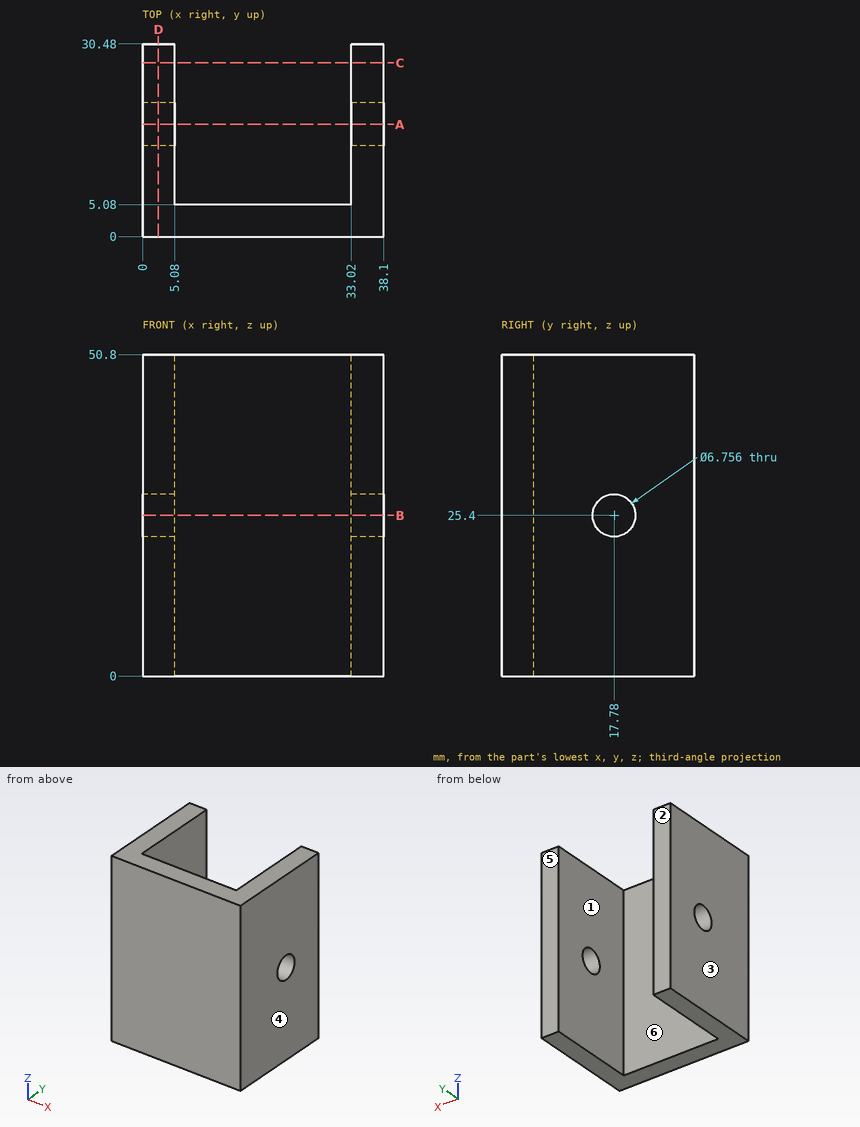
Study the drawing (mm; zero at the part's minimum x, y, z) and answer. A direction names the side the tool comes from. Round coordinates to 2 decimals unless told otherwise and drop trailing zeros. Write each loop counter-clockwise with the first axis right and the second up, starting at its lowest first coordinate (ties: lowest second). Pieces come first, ordered by that corner, then holes. Notation, with made-up numbers: (-30.75, -22.75) - (0.25, -22.75) arc R26 cw to (0.25, -7.75) - close; hole circle Ø2 at (79, 1.5). An arc over 180 degrees is marked (long way). Return JSON: item names as keys, results as strings. Group by question number.
Q1. The part is cut by section C-C on y = 27.5. Write down the section's boundary in (x, z), then the cut area to 3 significant figures.
Q2. Find the intervals of material crossed by L1, parallel to X at y = 23.5, z = 11.5; L2, parallel to Y at x = 3, z = 25.4; L3, parallel to Z at x = 37, y = 17.78, in increasing order.
Q3. The part is cut by section A-A on y = 17.78. Write down the section's boundary in (x, z).
Q4. This flat-tipped pin is pushed along its axis until it touches: pin 1 Ø14 at (x, z) = (25, 15) entering from +Y. Where does it stop, or does it pass through?
Q5. For the marked faces 1 and 2, determine the directions among +Z, -Z, +X, -X, +Y, -Y from which every point of the face is accessible in a straight line to the end or side of a thin tool.
Q6. The part is cut by section D-D on x = 2.5. Write down the section's boundary in (y, z), then the cut area to 3 significant figures.
Q7. The mould has two halves that part along X. Classify the marked faces 3, 4, 5 and 6: released by +X, released by -X, zero draft, split by the parting line, or undercut.
Q8. The part is cut by section B-B on z = 25.4. Write down the section's boundary in (x, y).
Solved:
{
 "1": {"outline": "(0, 0) - (5.08, 0) - (5.08, 50.8) - (0, 50.8) - close; (33.02, 0) - (38.1, 0) - (38.1, 50.8) - (33.02, 50.8) - close", "area": "516 mm²"},
 "2": {"L1": "0 to 5.08, 33.02 to 38.1", "L2": "0 to 14.4, 21.16 to 30.48", "L3": "0 to 22.02, 28.78 to 50.8"},
 "3": {"outline": "(0, 0) - (5.08, 0) - (5.08, 22.02) - (0, 22.02) - close; (0, 28.78) - (5.08, 28.78) - (5.08, 50.8) - (0, 50.8) - close; (33.02, 0) - (38.1, 0) - (38.1, 22.02) - (33.02, 22.02) - close; (33.02, 28.78) - (38.1, 28.78) - (38.1, 50.8) - (33.02, 50.8) - close"},
 "4": {"pin 1": "y = 5.08"},
 "5": {"face 1": "+Z, -Z, +Y", "face 2": "+Z, -Z, +X, -X, +Y"},
 "6": {"outline": "(0, 0) - (30.48, 0) - (30.48, 50.8) - (0, 50.8) - close; hole circle Ø6.76 at (17.78, 25.4)", "area": "1,510 mm²"},
 "7": {"face 3": "released by -X", "face 4": "released by +X", "face 5": "zero draft", "face 6": "undercut"},
 "8": {"outline": "(0, 0) - (38.1, 0) - (38.1, 14.4) - (33.02, 14.4) - (33.02, 5.08) - (5.08, 5.08) - (5.08, 14.4) - (0, 14.4) - close; (0, 21.16) - (5.08, 21.16) - (5.08, 30.48) - (0, 30.48) - close; (33.02, 21.16) - (38.1, 21.16) - (38.1, 30.48) - (33.02, 30.48) - close"}
}
